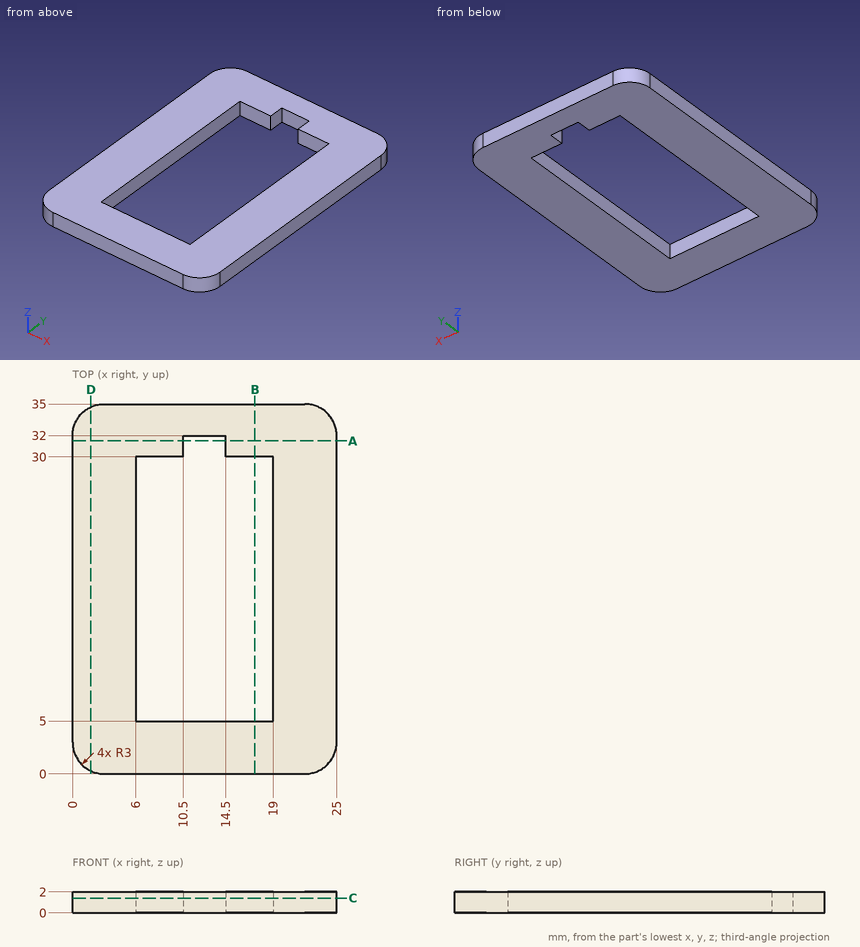
Check sheet for the drawn part. Datum: minimum x, y, z corner. Units: mm. Coordinates: 2 decimals unless noted, no trailing zeros. Loops run counter-clockwise (first coordinate to the right, second up) from the corner with the lowest first, then second, coordinate; pieces in that order, holes last. Notation, with made-up numbers: (72, 71.5) -> (89, 71.5) arc R14 ccw to (89, 75.5) -> close; hole circle Ø10 at (13.5, 74.25). An arc over 180 degrees is marked (long way). Answer as a JSON object with one key per item and string values. Group by question number.
Item 1: Sectioned sample at B-B on x = 17.25. Record the boundary of the cut face in (y, z), plus the area to 3 significant figures.
Item 2: Sectioned sample at A-A on y = 31.5. Record the boundary of the cut face in (x, z).
Item 3: Sectioned sample at D-D on x = 1.75. Record the boundary of the cut face in (y, z), plus the area to 3 significant figures.
Item 4: Sectioned sample at C-C on z = 1.4. Record the boundary of the cut face in (x, y).
Item 5: Depth check by flat-ended pin: pin 1 (0.6 mm diameter, centred on y = 30.5, z = 0.5, fed in from -X). Enter the tip coordinate at first touch or a pass-through.
Item 6: Scan lines: probe 1 along Y at (x, z) = (7.5, 0.6); probe 2 along X at (y, z) = (10, 1.8); probe 3 along X at (y, z) = (31.5, 1.8). Record each from-to range of solid material in increasing order.
Evaluation:
{
 "1": {"outline": "(0, 0) -> (5, 0) -> (5, 2) -> (0, 2) -> close; (30, 0) -> (35, 0) -> (35, 2) -> (30, 2) -> close", "area": "20.0 mm²"},
 "2": {"outline": "(0, 0) -> (10.5, 0) -> (10.5, 2) -> (0, 2) -> close; (14.5, 0) -> (25, 0) -> (25, 2) -> (14.5, 2) -> close"},
 "3": {"outline": "(0.27, 0) -> (34.73, 0) -> (34.73, 2) -> (0.27, 2) -> close", "area": "68.9 mm²"},
 "4": {"outline": "(0, 3) arc R3 ccw to (3, 0) -> (22, 0) arc R3 ccw to (25, 3) -> (25, 32) arc R3 ccw to (22, 35) -> (3, 35) arc R3 ccw to (0, 32) -> close; hole (6, 5) -> (19, 5) -> (19, 30) -> (14.5, 30) -> (14.5, 32) -> (10.5, 32) -> (10.5, 30) -> (6, 30) -> close"},
 "5": {"pin 1": "stops at x = 0"},
 "6": {"probe 1": "y = 0 to 5, 30 to 35", "probe 2": "x = 0 to 6, 19 to 25", "probe 3": "x = 0 to 10.5, 14.5 to 25"}
}
